Here's how the part is built. I have some questions about the finished solid (model axes, mm). Face numbers are marked on the shaded views. Give positions to 0.01 mm unless a question says otherwise; leave off trailing zeros. Loops run counter-clockwise (first coordinate to the right, second up) from the corner with the lowest first, then second, coordinate; pieces in that order, holes last.
Q1. Suppose I cut it at D-D (x = -24). List the corners of the cut face in (y, z) for me.
Q2. Suppose I cut it at A-A (y = 44). List the corners of the cut face in (x, z) for me, and give its area (4 significant figures).
Q3. Thinking about a two-plate mould opening in Z: for the marked faces 1, 2 and 3, which applies, pulls with the +Z half, pulls with the -Z half, needs draft (parallel to the pull), parting line crosses it, or undercut?
Q4. Suppose I cut it at B-B (z = -19). List the corners of the cut face in (x, y) for me, and give its area (3 significant figures).
Q5. Suppose I cut it at C-C (x = 17). List the corners of the cut face in (y, z) for me.
Q6. I need wall thicknesses on probe 1 along X at (y, z) = (1.9, 19); probe 2 along Z at (x, y) = (-24, 3.75); probe 3 along Z at (x, y) = (-8.5, 1.9). Which ranges of each line are inside material? Lowest first, please.
Q7. I'm going to push flat-ended pins straight in: P1, Ø2, axis at x = 28.5, z = 19, coming from the -Y side; P2, Ø3, axis at x = -24.5, z = 7, coming from the +Y side; P3, Ø1.8, axis at x = 19.5, z = -31.5, coming from the -Y side; P4, Ø2, axis at x = 8, y = 73, coming from the -Z side. Where does each tip first touch, or does it pass through?
Autodesk Inventor part; units mm, degrees
ref_plane "YZ Plane" through (0, 0, 0) normal (1, 0, 0) x (0, 1, 0)
ref_plane "XZ Plane" through (0, 0, 0) normal (0, 1, 0) x (-1, 0, 0)
ref_plane "XY Plane" through (0, 0, 0) normal (0, 0, 1) x (1, 0, 0)
sketch "Sketch1" plane through (0, 0, 0) normal (0, 1, 0) x (-1, 0, 0)
  line L0 (-30, 34) -> (30, 34)
  line L1 (30, 34) -> (30, -34)
  line L2 (30, -34) -> (-30, -34)
  line L3 (-30, -34) -> (-30, 34)
  line L4 (-30, 34) -> (30, -34) construction
  line L5 (30, 34) -> (-30, -34) construction
  line L6 (30, 34) -> (30, 19)
  line L7 (-30, -34) -> (-23, -34)
  line L8 (-30, -34) -> (8.5, -34)
  circle A0 centre (8.5, -31.5) radius 1.5
  circle A1 centre (-19.5, -31.5) radius 1.5
  circle A2 centre (-19.5, -31.5) radius 1.5
  circle A3 centre (24, 19) radius 1.5
  line L9 (24, 19) -> (0, 19)
  line L10 (0, 19) -> (0, 0)
  line L11 (0, 0) -> (8.5, -31.5)
  line L12 (8.5, -31.5) -> (0, -31.5)
  line L13 (-19.5, -31.5) -> (-19.5, 0)
  line L14 (-19.5, 0) -> (0, 0)
  line L15 (30, 34) -> (37, 34)
  line L16 (-37, -34) -> (37, -34)
  line L17 (37, -34) -> (37, 34)
  line L18 (37, 34) -> (-37, 34)
  line L19 (-37, 34) -> (-37, -34)
  line L20 (-37, -34) -> (37, 34) construction
  line L21 (37, -34) -> (-37, 34) construction
  dimension "d0" = 60
  dimension "d1" = 68
  dimension "d3" = 7
  dimension "d5" = 3
  dimension "d6" = 3
  dimension "d7" = 3
  dimension "d10" = 7
  dimension "d11" = 31.5
  dimension "d12" = 19.5
  dimension "d13" = 90
  dimension "d14" = 32.6267
  dimension "d15" = 8.5
  dimension "d16" = 24
extrude "Extrusion1" add sketch "Sketch1" along normal blind 6
sketch "Sketch2" plane through (0, 6, 0) normal (0, 1, 0) x (1, 0, 0)
  circle A0 centre (-24, -19) radius 1.5
  circle A1 centre (19.5, 31.5) radius 1.5
  circle A2 centre (-8.5, 31.5) radius 1.5
  line L0 (37, 34) -> (-37, 34)
  line L1 (-37, 34) -> (-37, -34)
  line L2 (-37, -34) -> (37, -34)
  line L3 (37, -34) -> (37, 34)
  line L4 (-37, 34) -> (-37, -34)
  line L5 (-33.5, 34) -> (-30, 34)
  line L6 (-30, 34) -> (-30, 27)
  line L7 (-30, 27) -> (-37, 27)
  line L8 (-37, 27) -> (-37, 30.5)
  line L9 (-37, 30.5) -> (-33.5, 34)
  line L10 (37, 34) -> (-37, 34)
  line L11 (-37, -34) -> (-30, -34)
  line L12 (-30, -34) -> (-30, -27)
  line L13 (-30, -27) -> (-37, -27)
  line L14 (-37, -27) -> (-37, -30.5)
  line L15 (-37, -34) -> (37, -34)
  line L16 (33.5, -34) -> (30, -34)
  line L17 (30, -34) -> (30, -27)
  line L18 (30, -27) -> (37, -27)
  line L19 (37, -27) -> (37, -30.5)
  line L20 (33.5, 34) -> (30, 34)
  line L21 (30, 34) -> (30, 27)
  line L22 (30, 27) -> (37, 27)
  line L23 (37, 27) -> (37, 30.5)
  line L24 (-30, -34) -> (-33.5, -34)
  line L25 (-33.5, -34) -> (-37, -30.5)
  line L26 (-37, -30.5) -> (-37, -27)
  line L27 (33.5, -34) -> (37, -30.5)
  line L28 (37, -34) -> (37, 34)
  line L29 (37, -30.5) -> (37, -27)
  line L30 (33.5, -34) -> (30, -34)
  line L31 (37, 27) -> (37, 30.5)
  line L32 (37, 30.5) -> (33.5, 34)
  line L33 (33.5, 34) -> (30, 34)
  point P0 (0, 0)
  dimension "d19" = 7
  dimension "d20" = 7
  dimension "d21" = 7
  dimension "d22" = 7
  dimension "d23" = 7
  dimension "d24" = 7
  dimension "d25" = 7
  dimension "d26" = 7
  dimension "d27" = 3.5
extrude "Extrusion2" add sketch "Sketch2" along normal blind 60 contours L32 L3 L22 L21 L0 | L6 L7 L1 L9 L0 | L3 L27 L2 L17 L18 | L13 L12 L2 L25 L1
sketch "Sketch3" plane through (0, 66, 0) normal (0, 1, 0) x (1, 0, 0)
  line L0 (37, 30.5) -> (33.5, 34)
  line L1 (33.5, 34) -> (30, 34)
  line L2 (30, 34) -> (30, 27)
  line L3 (30, 27) -> (37, 27)
  line L4 (37, 27) -> (37, 30.5)
  line L5 (37, -30.5) -> (37, -27)
  line L6 (37, -27) -> (30, -27)
  line L7 (30, -27) -> (30, -34)
  line L8 (30, -34) -> (33.5, -34)
  line L9 (33.5, -34) -> (37, -30.5)
  line L10 (-30, -34) -> (-30, -27)
  line L11 (-30, -27) -> (-37, -27)
  line L12 (-37, -27) -> (-37, -30.5)
  line L13 (-37, -30.5) -> (-33.5, -34)
  line L14 (-33.5, -34) -> (-30, -34)
  line L15 (-30, 27) -> (-30, 34)
  line L16 (-33.5, 34) -> (-37, 30.5)
  line L17 (-37, 30.5) -> (-37, 27)
  line L18 (-37, 27) -> (-30, 27)
  line L19 (-30, 27) -> (-30, 34)
  line L20 (-30, 34) -> (-33.5, 34)
  line L21 (-37, 34) -> (-30, 34)
  line L22 (-30, 34) -> (-30, -34)
  line L23 (-30, -34) -> (-37, -34)
  line L24 (-37, -34) -> (-37, 34)
  line L25 (30, 34) -> (30, 27)
  line L26 (37, -34) -> (30, -34)
  line L27 (30, -34) -> (30, 34)
  line L28 (30, 34) -> (37, 34)
  line L29 (37, 34) -> (37, -34)
  line L30 (-30, -34) -> (-30, -27)
  line L31 (37, -27) -> (30, -27)
  line L32 (-30, -34) -> (30, -34)
  line L33 (30, -34) -> (30, -27)
  line L34 (30, -27) -> (-30, -27)
  line L35 (-30, -27) -> (-30, -34)
  point P0 (0, 0)
extrude "Extrusion3" add sketch "Sketch3" along normal blind 8
sketch "Sketch4" plane through (37, 0, -34) normal (0, 0, -1) x (-1, 0, 0)
  line L0 (0, 66) -> (0, 74)
  line L1 (0, 74) -> (7, 74)
  line L2 (7, 74) -> (7, 66)
  line L3 (7, 66) -> (0, 66)
  line L4 (0, 66) -> (0, 74)
  line L5 (74, 6) -> (74, 66)
  line L6 (74, 66) -> (67, 66)
  line L7 (67, 66) -> (67, 74)
  line L8 (67, 74) -> (74, 74)
  line L9 (74, 74) -> (74, 66)
  line L10 (7, 66) -> (7, 69)
  line L11 (7, 66) -> (7, 74)
  line L12 (7, 69) -> (3.5, 69)
  line L13 (3.5, 69) -> (3.5, 72)
  line L14 (3.5, 72) -> (7, 72)
  line L15 (7, 72) -> (7, 74)
  line L16 (3.5, 72) -> (7, 72)
  line L17 (7, 72) -> (7, 69)
  line L18 (7, 69) -> (3.5, 69)
  line L19 (3.5, 69) -> (3.5, 72)
  line L20 (67, 6) -> (67, 66)
  line L21 (67, 66) -> (67, 69)
  line L22 (67, 66) -> (67, 74)
  line L23 (67, 69) -> (70.5, 69)
  line L24 (70.5, 69) -> (70.5, 72)
  line L25 (70.5, 72) -> (67, 72)
  line L26 (67, 72) -> (67, 69)
  line L27 (7, 72) -> (67, 72)
  line L28 (67, 72) -> (67, 69)
  line L29 (67, 69) -> (7, 69)
  line L30 (7, 69) -> (7, 72)
  point P0 (37, 0)
  dimension "d32" = 3
  dimension "d33" = 3
  dimension "d34" = 3
  dimension "d35" = 3.5
  dimension "d36" = 3
extrude "Extrusion4" cut sketch "Sketch4" against normal blind 64.5 contours L12 L13 L14 L2 | L2 L27 L7 L29 | L7 L25 L24 L23
sketch "Sketch5" plane through (37, 0, 34) normal (1, 0, 0) x (0, 0, -1)
  line L0 (0, 0) -> (0, 6)
  line L1 (0, 0) -> (5.1764, -19.3185)
  line L2 (0, 0) -> (20, 0) construction
  line L3 (5.1764, -19.3185) -> (25.1764, -19.3185)
  line L4 (5.1764, -19.3185) -> (25.1764, -19.3185) construction
  line L5 (25.1764, -19.3185) -> (34, 0)
  line L6 (29.3317, -3) -> (23.2485, -16.3185)
  line L7 (23.2485, -16.3185) -> (7.4784, -16.3185)
  line L8 (7.4784, -16.3185) -> (3.9097, -3)
  line L9 (3.9097, -3) -> (20, -3)
  line L10 (20, -3) -> (29.3317, -3)
  dimension "d39" = 20
  dimension "d40" = 75
  dimension "d41" = 20
  dimension "d42" = 0
  dimension "d43" = 3
sketch "Sketch6" plane through (37, 0, 34) normal (1, 0, 0) x (0, 0, -1)
  line L0 (68, 0) -> (68, 6)
  line L1 (68, 0) -> (28, 0)
  line L2 (28, 0) -> (28, -13)
  line L3 (28, -13) -> (68, -13)
  line L4 (66, -11) -> (30, -11)
  line L5 (30, -11) -> (30, -2)
  line L6 (30, -2) -> (66, -2)
  line L7 (68, -13) -> (68, -11)
  line L8 (68, -2) -> (68, 0)
  line L9 (66, -11) -> (68, -11)
  line L10 (66, -2) -> (68, -2)
  point P0 (34, 0)
  dimension "d44" = 40
  dimension "d45" = 13
  dimension "d46" = 2
properties part number "Main_Body_Wheel"
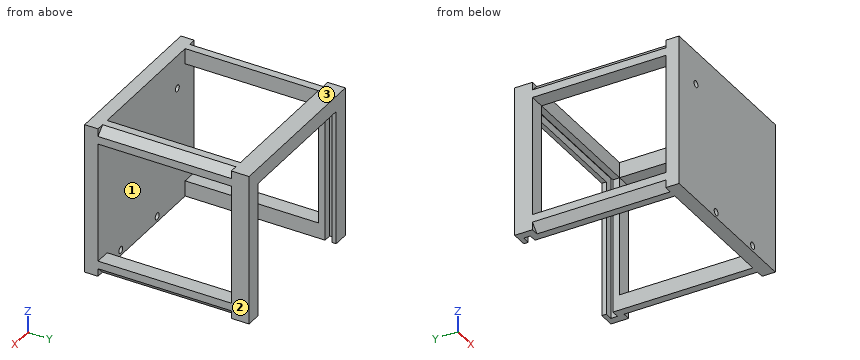
Solutions:
1. outline: (0, -34) - (6, -34) - (6, 17.5) - (0, 17.5) - close; (0, 20.5) - (6, 20.5) - (6, 34) - (0, 34) - close; (66, 27) - (69, 27) - (69, 30.5) - (72, 30.5) - (72, 27) - (74, 27) - (74, 34) - (66, 34) - close
2. outline: (-37, -30.5) - (-33.5, -34) - (-30, -34) - (-30, -27) - (-37, -27) - close; (-37, 27) - (-30, 27) - (-30, 34) - (-33.5, 34) - (-37, 30.5) - close; (30, -34) - (33.5, -34) - (37, -30.5) - (37, -27) - (30, -27) - close; (30, 27) - (37, 27) - (37, 30.5) - (33.5, 34) - (30, 34) - close
2. area: 171.5 mm2
3. face 1: undercut
3. face 2: needs draft
3. face 3: pulls with the +Z half
4. outline: (-37, 0) - (37, 0) - (37, 6) - (-37, 6) - close; (-37, 66) - (-30, 66) - (-30, 69) - (-33.5, 69) - (-33.5, 72) - (-30, 72) - (-30, 74) - (-37, 74) - close; (30, 66) - (37, 66) - (37, 74) - (30, 74) - (30, 72) - (33.5, 72) - (33.5, 69) - (30, 69) - close
4. area: 535 mm2
5. outline: (0, -34) - (6, -34) - (6, 34) - (0, 34) - close; (66, 27) - (69, 27) - (69, 30.5) - (72, 30.5) - (72, 27) - (74, 27) - (74, 34) - (66, 34) - close
6. probe 1: x = -37 to -25.5, -22.5 to 37
6. probe 2: z = -34 to 17.5, 20.5 to 34
6. probe 3: z = -34 to -33, -30 to 34
7. P1: stops at y = 0
7. P2: stops at y = 6
7. P3: passes through
7. P4: stops at z = 27
